Geometry check sheet. Reference: the model listing, model coordinates, mm. Face numbers are marked on the shaded views. Round coordinates to 2 decimals unless told otherwise and drop trailing zeros. Order: outer loops, then holes, each group sorted by start corner. A loop starts at its lowest first (then second) coordinate and runs counter-clockwise, first axis right, second up. Notation, with made-up numbers: (73.25, 16.5) - (126.25, 16.5) arc R10 ccw to (126.25, 28.5) - close; hole circle Ø2 at (-13.5, -9). An arc over 180 degrees is marked (long way). Write each question's results on one line, items separated by ' | '.
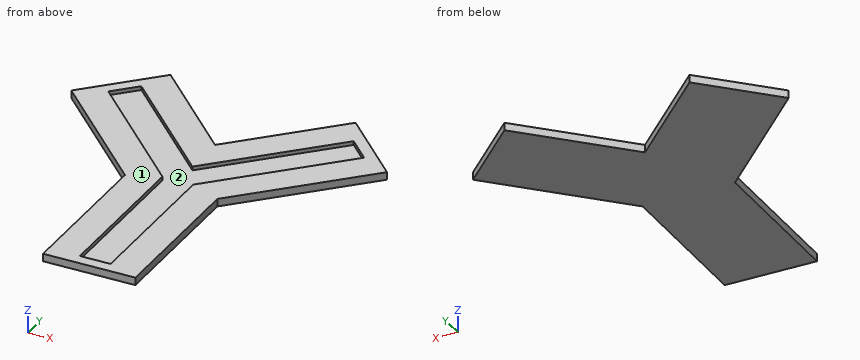
```python
from build123d import *

# Parameters (mm, degrees)
F1_DEPTH  = 43
F6_DEPTH  = 43
F8_DEPTH  = 43
F10_DEPTH = 43
F12_DEPTH = 43
F14_DEPTH = 43
F15_W     = 24
F15_H     = 2
F16_DEPTH = 3
F17_W     = 24
F17_H     = 2
F18_DEPTH = 3
F19_W     = 24
F19_H     = 2
F20_DEPTH = 3


with BuildPart() as f1:
    # F0 (on Front) → F1 (new body)
    with BuildSketch(Plane.XZ):
        Polygon((4, 0), (0, 0), (-4, 0), (-4, 1), (-12, 1), (-12, -1), (12, -1), (12, 1), (4, 1), align=None)
    extrude(amount=F1_DEPTH)

    # F5 (on face) → F6 (join)
    with BuildSketch(Plane(origin=(0, 0, 0), x_dir=(-0.7071067812, -0.7071067812, 0), z_dir=(-0.7071067812, 0.7071067812, 0))):
        Polygon((4, 0), (0, 0), (-4, 0), (-4, 1), (-12, 1), (-12, -1), (12, -1), (12, 1), (4, 1), align=None)
    extrude(amount=F6_DEPTH)

    # F7 (on face) → F8 (join)
    with BuildSketch(Plane(origin=(0, 0, 0), x_dir=(-0.7071067812, 0.7071067812, 0), z_dir=(0.7071067812, 0.7071067812, 0))):
        Polygon((4, 0), (0, 0), (-4, 0), (-4, 1), (-12, 1), (-12, -1), (12, -1), (12, 1), (4, 1), align=None)
    extrude(amount=F8_DEPTH)

    # F9 (on face) → F10 (cut)
    with BuildSketch(Plane.XZ.offset(43)):
        Polygon((-4, 0), (0, 0), (4, 0), (4, 1), (-4, 1), align=None)
    extrude(amount=-F10_DEPTH, mode=Mode.SUBTRACT)

    # F11 (on face) → F12 (cut)
    with BuildSketch(Plane(origin=(-30.405591591, 30.405591591, 0), x_dir=(-0.7071067812, -0.7071067812, 0), z_dir=(-0.7071067812, 0.7071067812, 0))):
        Polygon((-4, 0), (0, 0), (4, 0), (4, 1), (-4, 1), align=None)
    extrude(amount=-F12_DEPTH, mode=Mode.SUBTRACT)

    # F13 (on face) → F14 (cut)
    with BuildSketch(Plane(origin=(30.405591591, 30.405591591, 0), x_dir=(-0.7071067812, 0.7071067812, 0), z_dir=(0.7071067812, 0.7071067812, 0))):
        Polygon((-4, 0), (0, 0), (4, 0), (4, 1), (-4, 1), align=None)
    extrude(amount=-F14_DEPTH, mode=Mode.SUBTRACT)

    # F15 (on face) → F16 (join)
    with BuildSketch(Plane.XZ.offset(43)):
        Rectangle(F15_W, F15_H)
    extrude(amount=F16_DEPTH)

    # F17 (on face) → F18 (join)
    with BuildSketch(Plane(origin=(-30.405591591, 30.405591591, 0), x_dir=(-0.7071067812, -0.7071067812, 0), z_dir=(-0.7071067812, 0.7071067812, 0))):
        Rectangle(F17_W, F17_H)
    extrude(amount=F18_DEPTH)

    # F19 (on face) → F20 (join)
    with BuildSketch(Plane(origin=(30.405591591, 30.405591591, 0), x_dir=(-0.7071067812, 0.7071067812, 0), z_dir=(0.7071067812, 0.7071067812, 0))):
        Rectangle(F19_W, F19_H)
    extrude(amount=F20_DEPTH)


solid = f1.part
```
(1) Section check B-B (y = 23). Record the cut outline in (x, z).
Answers follow:
outline: (-39.97, -1) - (-6.03, -1) - (-6.03, 1) - (-17.34, 1) - (-17.34, 0) - (-28.66, 0) - (-28.66, 1) - (-39.97, 1) - close; (6.03, -1) - (39.97, -1) - (39.97, 1) - (28.66, 1) - (28.66, 0) - (17.34, 0) - (17.34, 1) - (6.03, 1) - close
(2) Section check C-C (x = -8.5). Record the cut outline in (y, z), then the cut area to 3 significant figures.
Answers follow:
outline: (-46, -1) - (25.47, -1) - (25.47, 1) - (14.16, 1) - (14.16, 0) - (2.84, 0) - (2.84, 1) - (-46, 1) - close | area: 132 mm²
(3) Draft check along X on the marked faces 1 and 2. Enter one of: released by +X, released by -X, zero draft, split by the parting line, or undercut.
Answers follow:
face 1: zero draft | face 2: undercut
(4) Section check D-D (y = -34). Record the cut outline in (x, z), then the cut area to 3 significant figures.
Answers follow:
outline: (-12, -1) - (12, -1) - (12, 1) - (4, 1) - (4, 0) - (-4, 0) - (-4, 1) - (-12, 1) - close | area: 40.0 mm²
(5) Section check A-A (z = 0.55). Record the cut outline in (x, y).
Answers follow:
outline: (-41.01, 24.04) - (-12, -4.97) - (-12, -46) - (12, -46) - (12, -4.97) - (41.01, 24.04) - (24.04, 41.01) - (0, 16.97) - (-24.04, 41.01) - close; hole (-33.23, 27.58) - (-4, -1.66) - (-4, -43) - (4, -43) - (4, -1.66) - (33.23, 27.58) - (27.58, 33.23) - (0, 5.66) - (-27.58, 33.23) - close
(6) Material ranges on line 1 (X direction, y = -8, z = 0.4); line 2 (X direction, y = 16.5, z = 0.1); line 3 (X direction, y = 30, z = 0.2), recorded low to high.
Answers follow:
line 1: -12 to -4, 4 to 12 | line 2: -33.47 to -22.16, -10.84 to 10.84, 22.16 to 33.47 | line 3: -35.05 to -30.81, -24.34 to -13.03, 13.03 to 24.34, 30.81 to 35.05
(7) Depth check by flat-ended pin: pin 1 Ø1.5 at (x, y) = (-1, -29) entering from +Z; pin 2 Ø1 at (y, z) = (-1.5, -0.5) entering from +X; pin 3 Ø0.5 at (y, z) = (-21.5, 0.5) entering from -X. Enter the tip coordinate at first touch or a pass-through.
Answers follow:
pin 1: z = 0 | pin 2: x = 15.97 | pin 3: x = -12
